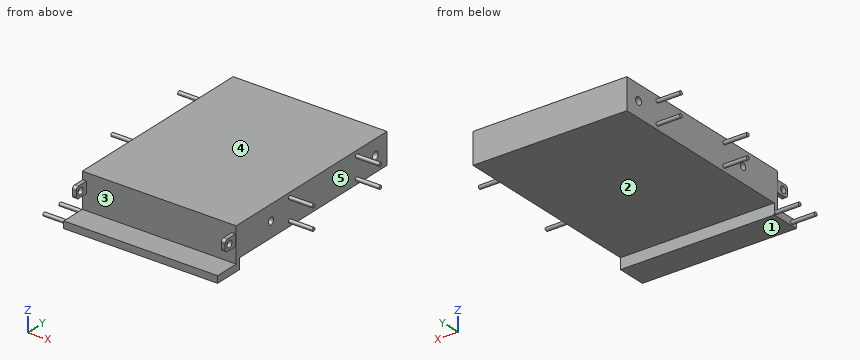
```python
from build123d import *

# Parameters (mm, degrees)
SKETCH1_W               = 127
SKETCH1_H               = 165.1
BOSS_EXTRUDE1_DEPTH     = 25.4
SKETCH3_R               = 2.921
CUT_EXTRUDE1_DEPTH      = 10.16
SKETCH4_R               = 1.4605
BOSS_EXTRUDE2_DEPTH     = 19.558
SKETCH5_R               = 1.4605
BOSS_EXTRUDE3_DEPTH     = 19.558
SKETCH6_W               = 3.173966583
SKETCH6_H               = 9.34053023
BOSS_EXTRUDE4_DEPTH     = 11.43
SKETCH7_R               = 2.794
CUT_EXTRUDE2_DEPTH      = 176.522086644
SKETCH8_R               = 3.187487877
CUT_EXTRUDE4_DEPTH      = 10.16
SKETCH11_R              = 1.4605
BOSS_EXTRUDE5_DEPTH     = 19.558
MIRROR6_COPY_1_SKETCH_R = 1.4605
MIRROR6_COPY_1_DEPTH    = 19.558
FILLET1_R               = 2.54
SKETCH15_W              = 127
SKETCH15_H              = 3.709069246
BOSS_EXTRUDE6_DEPTH     = 8.89
SKETCH16_W              = 127
SKETCH16_H              = 5.731432552
BOSS_EXTRUDE7_DEPTH     = 20.32
SKETCH17_R              = 1.4605
BOSS_EXTRUDE8_DEPTH     = 19.558
SKETCH18_R              = 1.4605
BOSS_EXTRUDE9_DEPTH     = 19.558


with BuildPart() as part:
    # Sketch1 → Boss-Extrude1 (new body)
    with BuildSketch(Plane.XY):
        Rectangle(SKETCH1_W, SKETCH1_H)
    extrude(amount=BOSS_EXTRUDE1_DEPTH)

    # Sketch3 → Cut-Extrude1 (cut)
    with BuildSketch(Plane.ZY.offset(63.5)):
        with Locations(Location((12.7, -44.45, 0), (0, 0, 270))):
            Circle(SKETCH3_R)
    cut_extrude1 = extrude(amount=-CUT_EXTRUDE1_DEPTH, mode=Mode.SUBTRACT)

    # Mirror1: Cut-Extrude1 across plane
    add(cut_extrude1.mirror(Plane(origin=(0, 0, 0), x_dir=(0, 0, 1), z_dir=(1, 0, 0))), mode=Mode.SUBTRACT)

    # Sketch4 → Boss-Extrude2 (add)
    with BuildSketch(Plane.ZY.offset(63.5)):
        with Locations(Location((3.9497, -23.876, 0), (0, 0, 90))):
            Circle(SKETCH4_R)
    boss_extrude2 = extrude(amount=BOSS_EXTRUDE2_DEPTH)

    # Sketch5 → Boss-Extrude3 (add)
    with BuildSketch(Plane.ZY.offset(63.5)):
        with Locations(Location((21.4503, -23.876, 0), (0, 0, 90))):
            Circle(SKETCH5_R)
    boss_extrude3 = extrude(amount=BOSS_EXTRUDE3_DEPTH)

    # Mirror2: Boss-Extrude2, Boss-Extrude3 across plane
    add(boss_extrude2.mirror(Plane(origin=(0, 0, 0), x_dir=(0, 0, 1), z_dir=(1, 0, 0))))
    add(boss_extrude3.mirror(Plane(origin=(0, 0, 0), x_dir=(0, 0, 1), z_dir=(1, 0, 0))))

    # Sketch6 → Boss-Extrude4 (add)
    with BuildSketch(Plane.XZ.offset(82.55)):
        with Locations((-61.405016708, 14.51369519)):
            Rectangle(SKETCH6_W, SKETCH6_H)
    boss_extrude4 = extrude(amount=BOSS_EXTRUDE4_DEPTH)

    # Mirror3: Boss-Extrude4 across plane
    add(boss_extrude4.mirror(Plane(origin=(0, 0, 0), x_dir=(0, 0, 1), z_dir=(1, 0, 0))))

    # Sketch7 → Cut-Extrude2 (cut, through all)
    with BuildSketch(Plane.ZY.offset(62.992)):
        with Locations((14.51369519, -89.281)):
            Circle(SKETCH7_R)
    extrude(amount=-CUT_EXTRUDE2_DEPTH, mode=Mode.SUBTRACT)

    # Sketch8 → Cut-Extrude4 (cut)
    with BuildSketch(Plane(origin=(63.5, 0, 0), x_dir=(0, 0, -1), z_dir=(1, 0, 0))):
        with Locations(Location((-12.7, 69.85, 0), (0, 0, 90))):
            Circle(SKETCH8_R)
    cut_extrude4 = extrude(amount=-CUT_EXTRUDE4_DEPTH, mode=Mode.SUBTRACT)

    # Sketch11 → Boss-Extrude5 (add)
    with BuildSketch(Plane(origin=(63.5, 0, 0), x_dir=(0, 0, -1), z_dir=(1, 0, 0))):
        with Locations(Location((-21.288830822, 49.276, 0), (0, 0, 270))):
            Circle(SKETCH11_R)
    boss_extrude5 = extrude(amount=BOSS_EXTRUDE5_DEPTH)

    # Mirror4: Boss-Extrude5 across plane
    add(boss_extrude5.mirror(Plane.XY.offset(12.7)))

    # Mirror6: Cut-Extrude4, Boss-Extrude5 across plane
    add(cut_extrude4.mirror(Plane(origin=(0, 0, 0), x_dir=(0, 0, 1), z_dir=(1, 0, 0))), mode=Mode.SUBTRACT)
    add(boss_extrude5.mirror(Plane(origin=(0, 0, 0), x_dir=(0, 0, 1), z_dir=(1, 0, 0))))

    # Mirror6 copy 1 sketch → Mirror6 copy 1 (add)
    with BuildSketch(Plane(origin=(-63.5, 0, 25.4), x_dir=(0, 0, 1), z_dir=(-1, 0, 0))):
        with Locations(Location((-21.288830822, 49.276, 0), (0, 0, 270))):
            Circle(MIRROR6_COPY_1_SKETCH_R)
    extrude(amount=MIRROR6_COPY_1_DEPTH)

    # Fillet1
    fillet1_edges = [part.edges().sort_by_distance(p)[0] for p in [
        (-61.405016709, -93.98, 9.843430075),
        (-61.405016709, -93.98, 19.183960305),
        (61.405016709, -93.98, 19.183960305),
        (61.405016709, -93.98, 9.843430075),
    ]]
    fillet(fillet1_edges, radius=FILLET1_R)

    # Sketch15 → Boss-Extrude6 (add)
    with BuildSketch(Plane(origin=(0, 0, 0), x_dir=(-1, 0, 0), z_dir=(0, 0, -1))):
        with Locations((0, -80.695465377)):
            Rectangle(SKETCH15_W, SKETCH15_H)
    extrude(amount=BOSS_EXTRUDE6_DEPTH)

    # Sketch16 → Boss-Extrude7 (add)
    with BuildSketch(Plane.XZ.offset(82.55)):
        with Locations((0, -6.024283724)):
            Rectangle(SKETCH16_W, SKETCH16_H)
    extrude(amount=BOSS_EXTRUDE7_DEPTH)

    # Sketch17 → Boss-Extrude8 (add)
    with BuildSketch(Plane.ZY.offset(63.5)):
        with Locations(Location((-6.35, -80.618930754, 0), (0, 0, 90))):
            Circle(SKETCH17_R)
    extrude(amount=BOSS_EXTRUDE8_DEPTH)

    # Sketch18 → Boss-Extrude9 (add)
    with BuildSketch(Plane.ZY.offset(63.5)):
        with Locations(Location((-6.35, -98.144930754, 0), (0, 0, 90))):
            Circle(SKETCH18_R)
    extrude(amount=BOSS_EXTRUDE9_DEPTH)


solid = part.part
```
Check sheet for the modelled part. Datum: model origin and axes. Units: mm. Face numbers are marked on the shaded views. A direction names the side the tool comes from. Round coordinates to 2 decimals unless told otherwise and drop trailing zeros. Write each loop counter-clockwise with the first axis right and the second up, starting at its lowest first coordinate (ties: lowest second). Pieces come first, ordered by that corner, then holes. Notation, with made-up numbers: (76.5, 52.25) -> (89.5, 52.25) arc R24 ccw to (89.5, 90.25) -> close; hole circle Ø1 at (40, 37). An arc over 180 degrees is marked (long way). One line per question, with ' | ' between items. Start each with the question number.
1. Release check for a two-part mould opening along X. For the marked faces 3, 4 and 5 record: +X half, -X half, draft (parallel to the pull), parting line (faces both ways), or undercut.
2. Sectioned sample at A-A, the plane y = 69.85. Record the cut outline in (x, z), then the cut area to 3 significant figures.
3. Sectioned sample at B-B, the plane x = -32. Record the cut outline in (y, z).
4. Sectioned sample at D-D, the plane y = 4.5. Record the cut outline in (x, z).
5. Sectioned sample at C-C, the plane x = 71. Record the cut outline in (y, z), then the cut area to 3 significant figures.
6. Set-up check for the marked faces 1 and 2: record each of +Z, -Z, +X, -X, +Y, -Y from which the full face is reachable in a straight line by a thin tool's end or side.
7. Scan lines: line 1 along Z through (x, y) = (-58.5, -44.45); line 2 along Y through (x, z) = (60, 13); line 3 along Z through (x, y) = (53.5, -32). Record each from-to range of solid material in increasing order. Write a range as from..to.
8. Depth check by flat-ended pin: pin 1 (1.9 mm diameter, centred on y = 71, z = 11.5, fed in from +X); pin 2 (6 mm diameter, centred on x = 39.5, z = 3, fed in from -Y); pin 3 (3.5 mm diameter, centred on x = 62, y = -88, fed in from +Z); pin 4 (4.5 mm diameter, centred on y = -89.28, z = 14.51, fed in from -X). Enter the tip coordinate at first touch or a pass-through.
Taken from the geometry:
1) face 3: undercut | face 4: draft | face 5: +X half
2) outline: (-63.5, 0) -> (63.5, 0) -> (63.5, 9.51) -> (53.34, 9.51) -> (53.34, 15.89) -> (63.5, 15.89) -> (63.5, 25.4) -> (-63.5, 25.4) -> (-63.5, 15.89) -> (-53.34, 15.89) -> (-53.34, 9.51) -> (-63.5, 9.51) -> close | area: 3,100 mm^2
3) outline: (-102.87, -8.89) -> (-78.84, -8.89) -> (-78.84, 0) -> (82.55, 0) -> (82.55, 25.4) -> (-82.55, 25.4) -> (-82.55, -3.16) -> (-102.87, -3.16) -> close
4) outline: (-63.5, 0) -> (63.5, 0) -> (63.5, 25.4) -> (-63.5, 25.4) -> close
5) outline: circle Ø2.92 at (-23.88, 3.95); circle Ø2.92 at (-23.88, 21.45); circle Ø2.92 at (49.28, 4.11); circle Ø2.92 at (49.28, 21.29) | area: 26.8 mm^2
6) face 1: -Z, +X, -X, +Y, -Y | face 2: -Z, +X, -X, +Y
7) line 1: z = 0..9.78, 15.62..25.4 | line 2: y = -93.98..-91.63, -86.93..-47.36, -41.54..66.68, 73.02..82.55 | line 3: z = 0..25.4
8) pin 1: stops at x = 53.34 | pin 2: stops at y = -82.55 | pin 3: stops at z = 19.18 | pin 4: passes through
